Answer from the drawing. Dimensions are ordinates in mm from the lowest x, y and z of the part. Coordinates: 2 decimals unless noted, no trailing zeros. Write each loop counter-clockwise with the first axis right and the second up, starting at its lowest first coordinate (ties: lowest second). Pieces come first, ordered by that corner, then holes. Notation, with made-up numbers: (-31, 53.25) -> (-7, 53.25) arc R18 ccw to (-7, 75.25) -> close; hole circle Ø9 at (46.5, -13). An arc over 180 degrees is marked (long way). Answer as a JSON object with one key per item and string values. Group by question number.
(1) Find section B-B (x = 192). Give the vertices of the cut face in (y, z).
(2) Flat-ended cylindrical pins translate along their axes: P1, Ø3, axis at x = 56, z = 6.5, coming from the +Y side; P2, Ø2.5, axis at x = 152, z = 18, coming from the +Y side; P3, Ø2, axis at x = 99, z = 1.5, coming from the +Y side. Find the tip coordinate at first contact, or state that the pin passes through.
(3) Find section C-C (y = 3). Give the vertices of the cut face in (x, z).
(4) Find section D-D (x = 167.5). Give the vertices of the cut face in (y, z), then the cut area to 3 significant figures.
(5) Straight lines are drawn through the part: L1, parallel to Z at x = 70, y = 31.5; L2, parallel to X at y = 12, z = 18 (1 decimal); L3, parallel to X at y = 33, z = 18.5. For each, find the intervals that lie inside material, in ascending order.
(6) Find section A-A (y = 19.25). Give the vertices of the cut face in (x, z), then the cut area to 3 significant figures.
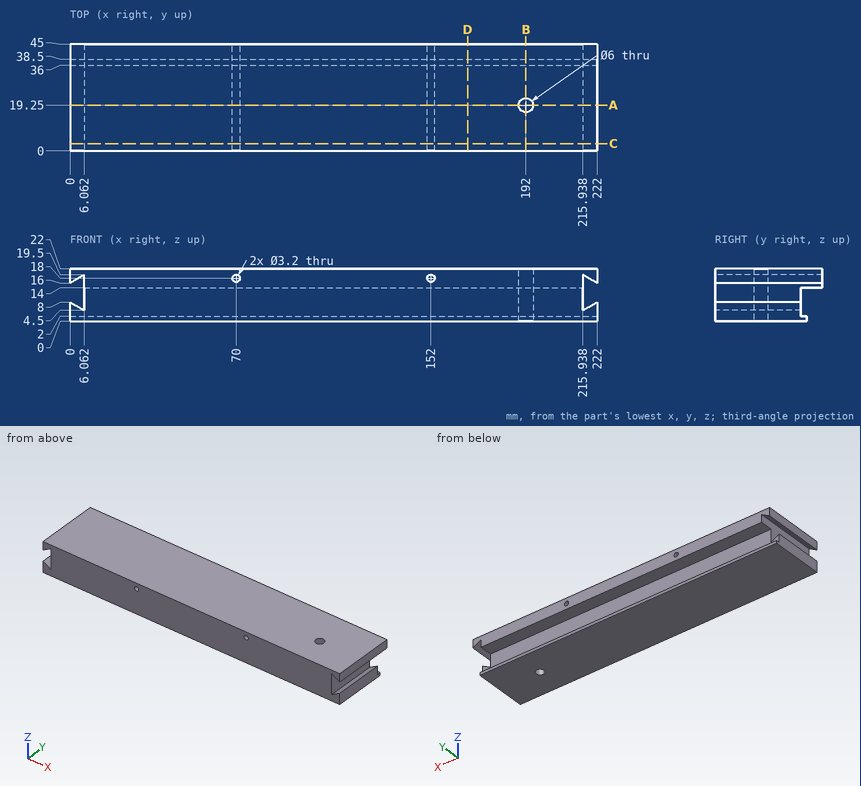
Results below:
{
 "1": {"outline": "(0, 0) -> (16.25, 0) -> (16.25, 22) -> (0, 22) -> close; (22.25, 0) -> (38.5, 0) -> (38.5, 2) -> (36, 2) -> (36, 14) -> (45, 14) -> (45, 22) -> (22.25, 22) -> close"},
 "2": {"P1": "stops at y = 36", "P2": "passes through", "P3": "stops at y = 38.5"},
 "3": {"outline": "(0, 0) -> (222, 0) -> (222, 8) -> (215.94, 4.5) -> (215.94, 19.5) -> (222, 16) -> (222, 22) -> (0, 22) -> (0, 16) -> (6.06, 19.5) -> (6.06, 4.5) -> (0, 8) -> close; hole circle Ø3.2 at (70, 18); hole circle Ø3.2 at (152, 18)"},
 "4": {"outline": "(0, 0) -> (38.5, 0) -> (38.5, 2) -> (36, 2) -> (36, 14) -> (45, 14) -> (45, 22) -> (0, 22) -> close", "area": "869 mm2"},
 "5": {"L1": "z = 0 to 16.4, 19.6 to 22", "L2": "x = 0 to 3.5, 6.1 to 68.4, 71.6 to 150.4, 153.6 to 215.9, 218.5 to 222", "L3": "x = 0 to 4.33, 6.06 to 68.48, 71.52 to 150.48, 153.52 to 215.94, 217.67 to 222"},
 "6": {"outline": "(0, 0) -> (189, 0) -> (189, 22) -> (0, 22) -> (0, 16) -> (6.06, 19.5) -> (6.06, 4.5) -> (0, 8) -> close; (195, 0) -> (222, 0) -> (222, 8) -> (215.94, 4.5) -> (215.94, 19.5) -> (222, 16) -> (222, 22) -> (195, 22) -> close; hole circle Ø3.2 at (70, 18); hole circle Ø3.2 at (152, 18)", "area": "4,600 mm2"}
}
